from build123d import *

# Parameters (mm, degrees)
SKETCH1_W           = 889
SKETCH1_H           = 889
SKETCH1_W_2         = 685.8
SKETCH1_H_2         = 685.8
BOSS_EXTRUDE1_DEPTH = 127
FILLET1_R           = 38.1
FILLET2_R           = 12.7
SKETCH2_W           = 101.6
SKETCH2_H           = 63.5
CUT_EXTRUDE1_DEPTH  = 128


with BuildPart() as part:
    # Sketch1 → Boss-Extrude1 (new body)
    with BuildSketch(Plane(origin=(0, 0, 0), x_dir=(1, 0, 0), z_dir=(0, 1, 0))):
        Rectangle(SKETCH1_W, SKETCH1_H)
        Rectangle(SKETCH1_W_2, SKETCH1_H_2, mode=Mode.SUBTRACT)
    extrude(amount=BOSS_EXTRUDE1_DEPTH)

    # Fillet1
    fillet1_edges = [part.edges().sort_by_distance(p)[0] for p in [
        (444.5, 63.5, -444.5),
        (444.5, 63.5, 444.5),
        (-444.5, 63.5, 444.5),
        (-444.5, 63.5, -444.5),
    ]]
    fillet(fillet1_edges, radius=FILLET1_R)

    # Fillet2
    fillet2_edges = [part.edges().sort_by_distance(p)[0] for p in [
        (-444.5, 0, 0),
        (-444.5, 127, 0),
        (0, 0, -444.5),
        (444.5, 0, 0),
        (0, 0, 444.5),
        (-433.340768363, 0, 433.340768363),
        (433.340768363, 0, 433.340768363),
        (433.340768363, 0, -433.340768363),
        (-433.340768363, 0, -433.340768363),
        (0, 127, -444.5),
        (0, 127, 444.5),
        (444.5, 127, 0),
        (-433.340768363, 127, 433.340768363),
        (433.340768363, 127, 433.340768363),
        (433.340768363, 127, -433.340768363),
        (-433.340768363, 127, -433.340768363),
    ]]
    fillet(fillet2_edges, radius=FILLET2_R)

    # Sketch2 → Cut-Extrude1 (cut, through all)
    with BuildSketch(Plane(origin=(0, 127, 0), x_dir=(1, 0, 0), z_dir=(0, 1, 0))):
        with Locations((393.7, 178.054)):
            Rectangle(SKETCH2_W, SKETCH2_H)
    extrude(amount=-CUT_EXTRUDE1_DEPTH, mode=Mode.SUBTRACT)


solid = part.part
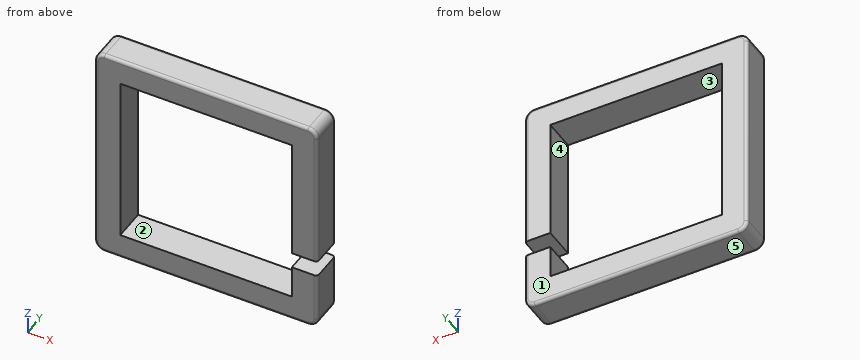
Can you work these out from the model? Positions are in its coordinate system, mm. Face numbers are marked on the shaded views. A direction names the side the tool comes from. Coordinates: 2 decimals unless noted, no trailing zeros. Write each loop counter-clockwise with the first axis right and the second up, starting at its lowest first coordinate (ties: lowest second). Pieces come first, ordered by that corner, then holes.
Q1. Imagine slicing it at B-B, the plane z = 201.5. List the corners of the cut face in (x, y) for me.
Results found:
outline: (-444.5, 12.7) arc R12.7 ccw to (-431.8, 0) - (-342.9, 0) - (-342.9, 127) - (-431.8, 127) arc R12.7 ccw to (-444.5, 114.3) - close; (342.9, 0) - (431.8, 0) arc R12.7 ccw to (444.5, 12.7) - (444.5, 114.3) arc R12.7 ccw to (431.8, 127) - (342.9, 127) - close
Q2. Imagine slicing it at A-A, the plane x = -313.5. List the corners of the cut face in (y, z) for me, plus the area to 3 significant figures.
Results found:
outline: (0, -431.8) arc R12.7 ccw to (12.7, -444.5) - (114.3, -444.5) arc R12.7 ccw to (127, -431.8) - (127, -342.9) - (0, -342.9) - close; (0, 342.9) - (127, 342.9) - (127, 431.8) arc R12.7 ccw to (114.3, 444.5) - (12.7, 444.5) arc R12.7 ccw to (0, 431.8) - close
area: 25,700 mm2
Q3. Please list where these lines run through material, in increasing order: L1, parallel to Z at x = 219, y = 67.5; L2, parallel to Z at x = -209, y = 10.
Results found:
L1: z = -444.5 to -342.9, 342.9 to 444.5
L2: z = -444.21 to -342.9, 342.9 to 444.21
Q4. If we mould it in two halves opening along X, with no side actions, what happens to the marked faces 3, 4 and 5? For each: +X half, -X half, draft (parallel to the pull), parting line (faces both ways), or undercut.
Results found:
face 3: undercut
face 4: undercut
face 5: draft
Q5. For P1, Ø5, axis at y = 112, z = -201.5, coming from the +X side, with a flat end and sliding along its axis, tell me the tip position at first contact or that it passes through.
Results found:
P1: stops at x = -342.9
Q6. Which directions (+Z, -Z, +X, -X, +Y, -Y) give clear straight access to the entire face, cutting with the end or side of a thin tool? Please do the marked faces 1 and 2.
Results found:
face 1: +Z, -Z, +X, -X, +Y
face 2: +Y, -Y
Q7. Imagine slicing it at C-C, the plane y = 55.5. List the corners of the cut face in (x, z) for me, plus the area to 3 significant figures.
Results found:
outline: (-444.5, -406.4) arc R38.1 ccw to (-406.4, -444.5) - (406.4, -444.5) arc R38.1 ccw to (444.5, -406.4) - (444.5, -209.8) - (342.9, -209.8) - (342.9, -342.9) - (-342.9, -342.9) - (-342.9, 342.9) - (342.9, 342.9) - (342.9, -146.3) - (444.5, -146.3) - (444.5, 406.4) arc R38.1 ccw to (406.4, 444.5) - (-406.4, 444.5) arc R38.1 ccw to (-444.5, 406.4) - close
area: 312,000 mm2
